Part model, mm, in its own coordinate system. Round coordinates to 2 decimals unless told otherwise and drop trailing zeros. Loops run counter-clockwise (first coordinate to the right, second up) from the corner with the lowest first, then second, coordinate; pieces in that order, holes last. Notation, with made-up numbers: (16, 63.25) -> (20, 63.25) arc R30 cw to (20, 101.25) -> close; hole circle Ø2 at (-24, 74.25). An arc over 180 degrees is marked (long way). Answer as CSV lines item,"result".
Solid Edge part; units mm, degrees
sketch "Sketch1" plane through (0, 0, 0) normal (0, -1, 0) x (1, 0, 0)
  circle A0 centre (0, 0) radius 31.5
extrude "Protrusion1" add sketch "Sketch1" against normal blind 18
sketch "Sketch2" plane through (0, 0, 0) normal (0, -1, 0) x (1, 0, 0)
  circle A0 centre (0, 0) radius 27.5
extrude "Cutout1" cut sketch "Sketch2" against normal through all
sketch "Sketch3" plane through (0, 0, 0) normal (0, 0, 1) x (1, 0, 0)
  line L0 (27.5, 0) -> (29.5, 18)
  line L1 (29.5, 18) -> (27.5, 18)
  line L2 (27.5, 18) -> (27.5, 0)
sketch3d "SweptCutout_4 path"
  arc A0 (27.5, 18, 0) -> (-13.75, 18, 23.8157) centre (0, 18, 0)
  arc A1 (-13.75, 18, 23.8157) -> (-13.75, 18, -23.8157) centre (0, 18, 0)
  arc A2 (-13.75, 18, -23.8157) -> (27.5, 18, 0) centre (0, 18, 0)
sweep "SweptCutout_4" cut profiles "Sketch3" path "SweptCutout_4 path"
sketch "Sketch4" plane through (0, 0, 0) normal (0, 0, 1) x (1, 0, 0)
  line L0 (31.5, 18) -> (29.5, 0)
  line L1 (29.5, 0) -> (31.5, 0)
  line L2 (31.5, 0) -> (31.5, 18)
sketch3d "SweptCutout_5 path"
  arc A0 (31.5, 0, 0) -> (-15.75, 0, 27.2798) centre (0, 0, 0)
  arc A1 (-15.75, 0, 27.2798) -> (-15.75, 0, -27.2798) centre (0, 0, 0)
  arc A2 (-15.75, 0, -27.2798) -> (31.5, 0, 0) centre (0, 0, 0)
sweep "SweptCutout_5" cut profiles "Sketch4" path "SweptCutout_5 path"
properties material "Aluminum, 1060"
Q1. Saw through at A-A, the plane z = 0. Write the cut outline in (x, y), then the cut area to 3 significant figures.
Geometry results:
outline,"(-31.5, 18) -> (-29.5, 0) -> (-27.5, 0) -> (-29.5, 18) -> close; (27.5, 0) -> (29.5, 0) -> (31.5, 18) -> (29.5, 18) -> close"
area,"72.0 mm2"
Q2. Saw through at C-C, the plane y = 15.75. Write the cut outline in (x, z) (3 decimals), then the cut area to 3 significant figures.
Geometry results:
outline,"circle Ø62.5 at (0, 0); hole (-14.625, -25.331) arc R29.25 ccw (long way) to (-14.625, 25.331) arc R29.25 ccw to start"
area,"380 mm2"
Q3. Drop flat-ended pins along their axis: P1, Ø1.5, axis at x = -1, y = 5.5, coming from the +Z side; P2, Ø3, axis at y = 13, z = -9, coming from the -X side; P3, Ø3, axis at x = -18.5, z = -15.5, coming from the -Y side; P4, Ø6, axis at x = -23, y = 7, coming from the +Z side. Give the stop position or say it passes through.
Geometry results:
P1,"z = 30.18"
P2,"x = -30.06"
P3,"through"
P4,"z = 22.77"
Q4. Saw through at B-B, the plane y = 9.25. Write the cut outline in (x, z), then the cut area to 3 significant figures.
Geometry results:
outline,"circle Ø61.06 at (0, 0); hole (-14.26, -24.71) arc R28.53 ccw (long way) to (-14.26, 24.71) arc R28.53 ccw to start"
area,"371 mm2"
Q5. Drill centre lines: line 1 along X through (y, z) = (13.5, 3); line 2 along Z through (x, y) = (-23, 1.5); line 3 along Z through (x, y) = (-14, 5.75). Where is each one in solid material? Low to high.
Geometry results:
line 1,"-30.85 to -28.84, 28.84 to 30.85"
line 2,"-18.74 to -15.38, 15.38 to 18.74"
line 3,"-26.69 to -24.41, 24.41 to 26.69"
